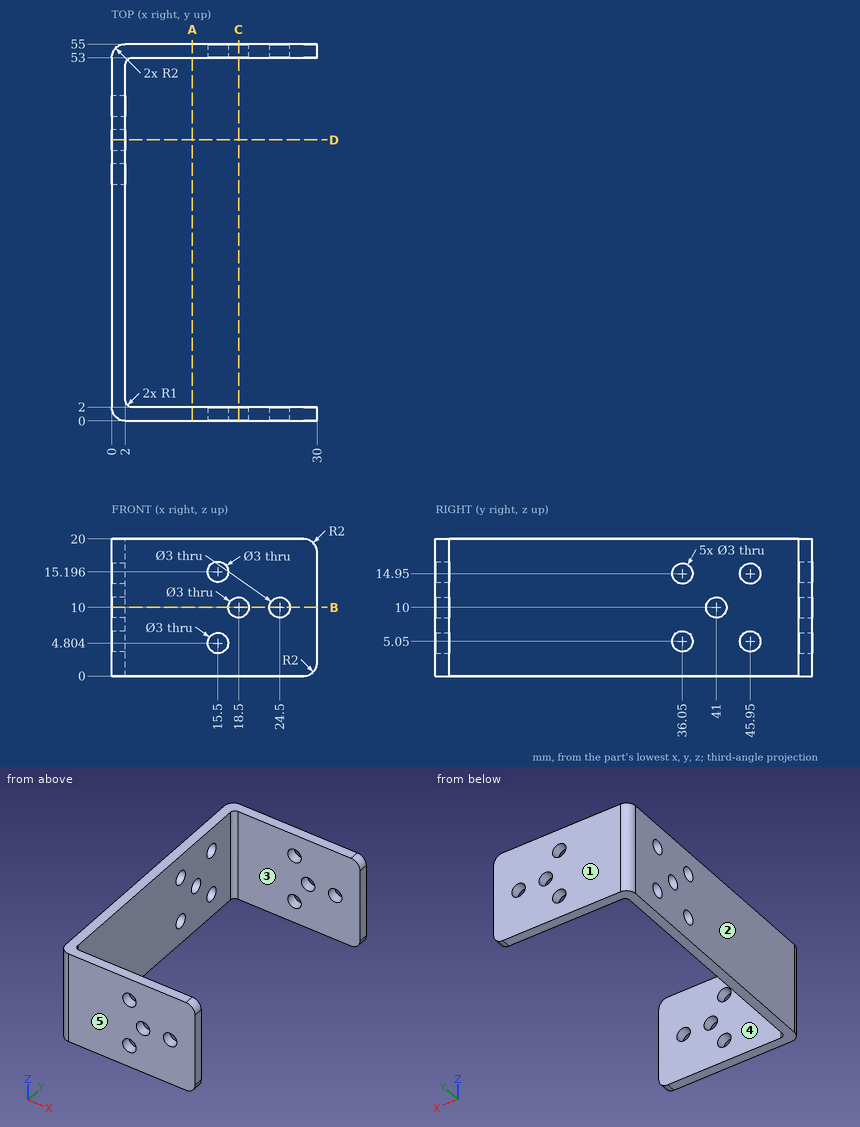
Answer from the drawing. Dimensions are ordinates in mm from the lowest x, y and z of the part. A direction names the side the tool comes from. Round coordinates to 2 decimals unless told otherwise and drop trailing zeros. Order: outer loops, then holes, each group sorted by start corner. A loop starts at its lowest first (then second) coordinate and runs counter-clockwise, first axis right, second up.
1) The part is cut by section D-D on y = 41. Write down the section's boundary in (x, z).
2) The part is cut by section C-C on x = 18.5. Write down the section's boundary in (y, z).
3) The part is cut by section B-B on z = 10. Give the number of separate pieces and of enclosed holes in the cut face, plus the area to 3 significant figures.
4) For the marked faces 4 and 5, determine the directions among +Z, -Z, +X, -X, +Y, -Y from which every point of the face is accessible in a straight line to the end or side of a thin tool.
5) The mould has two halves that part along Y. Classify the marked faces 1, 2 and 3: released by +Y, released by -Y, zero draft, split by the parting line, or undercut.
6) Straight lines are drawn through the part: L1, parallel to Z at x = 15.5, y = 1.5; L2, parallel to Z at x = 18.5, y = 53.6; L3, parallel to Y at x = 13, z = 18. For each, find the intervals that lie inside material, in ascending order.
7) Flat-ended cylindrical pins translate along their axes: pin 1 (6 mm diameter, centred on x = 19, z = 9.5, fed in from +Y); pin 2 (10 mm diameter, centred on y = 39, z = 10, fed in from +X). Find the tip coordinate at first contact, or state that the pin passes through.
8) The part is cut by section A-A on x = 11.75. Write down the section's boundary in (y, z), plus the area to 3 significant figures.
Resolved:
1. outline: (0, 0) - (2, 0) - (2, 8.5) - (0, 8.5) - close; (0, 11.5) - (2, 11.5) - (2, 20) - (0, 20) - close
2. outline: (0, 0) - (2, 0) - (2, 8.5) - (0, 8.5) - close; (0, 11.5) - (2, 11.5) - (2, 20) - (0, 20) - close; (53, 0) - (55, 0) - (55, 8.5) - (53, 8.5) - close; (53, 11.5) - (55, 11.5) - (55, 20) - (53, 20) - close
3. separate pieces: 6
3. enclosed holes: 0
3. area: 191 mm2
4. face 4: +Z, -Z, +X
4. face 5: +Z, -Z, +X, -X, -Y
5. face 1: released by +Y
5. face 2: zero draft
5. face 3: undercut
6. L1: z = 0 to 3.3, 6.3 to 13.7, 16.7 to 20
6. L2: z = 0 to 8.5, 11.5 to 20
6. L3: y = 0 to 2, 53 to 55
7. pin 1: stops at y = 55
7. pin 2: stops at x = 2
8. outline: (0, 0) - (2, 0) - (2, 20) - (0, 20) - close; (53, 0) - (55, 0) - (55, 20) - (53, 20) - close
8. area: 80.0 mm2
